For this review, take the finished solid that the model builds, in its own axes (mm). Face numbers are marked on the shaded views. A direction names the side the tool comes from. Coordinates: 2 decimals unless noted, no trailing zeros. Loops run counter-clockwise (first coordinate to the right, second up) from the corner with the lowest first, then second, coordinate; pieces in that order, holes last.
1. Take a section at A-A, the plane x = 1.5. State the section outline as (y, z) points, then the cut area to 3 significant figures.
2. Machinability: for the marked faces 4, 5 and 6, which of the approach directions +Z, -Z, +X, -X, +Y, -Y give a long, thin tool a straight path to every point of the face, cutting with its end or side? Answer none if there is none.
3. To check wall thickness, follow probe 1 along Z at (x, y) = (1.75, 0); probe 2 along Z at (x, y) = (3.75, 0); probe 3 along Y at (x, z) = (5.25, 2). State the ranges of each line that lie inside material, in increasing order.
4. Mouldability with a two-part tool opening along Y and no side actions: class the marked faces 1, 2 and 3 as pulls with the +Y half, pulls with the -Y half, needs draft (parallel to the pull), parting line crosses it, or undercut.
5. Clearance check with flat-ended pins moving along their axes: P1, Ø6, axis at x = 1, z = 11.5, coming from the -Y side; P2, Ø1.5, axis at x = -3.5, y = 13, coming from the -Z side; P3, Ø4, axis at x = 4.5, y = 12, coming from the -Z side; P4, Ø11, axis at y = -2.5, z = -0.5, coming from the -X side. State where each tip first meets the part, or that it passes through.
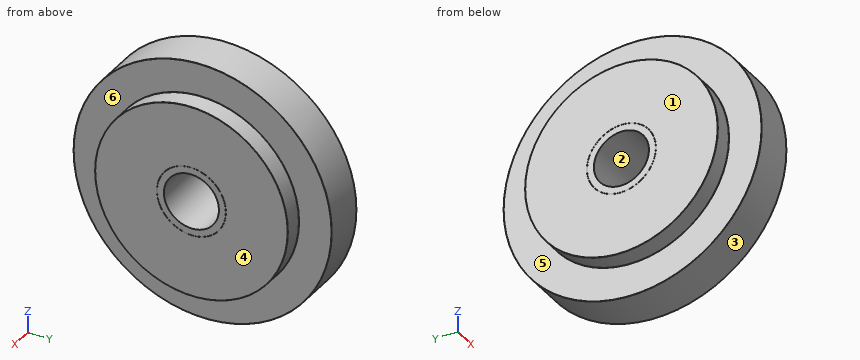
Autodesk Inventor part; units mm, degrees
ref_plane "to_bolt_XY" through (5.8, 0, 0) normal (1, 0, 0) x (0, 0, -1)
ref_plane "to_bolt_YZ" through (5.8, 0, 0) normal (0, 0, -1) x (0, 1, 0)
ref_plane "to_bolt_ZX" through (5.8, 0, 0) normal (0, 1, 0) x (1, 0, 0)
sketch "Sketch_1" plane through (0, 0, 0) normal (0, 0, 1) x (1, 0, 0)
  line L0 (5.8, 0) -> (-5.8, 0)
  line L1 (-5.8, 5.02) -> (-5.78, 5)
  line L2 (-5.78, 5) -> (5.78, 5)
  line L3 (5.78, 5) -> (5.8, 5.02)
  line L4 (5.8, 5.02) -> (5.8, 13.98)
  line L5 (5.8, 13.98) -> (5.78, 14)
  line L6 (5.78, 14) -> (3.081, 14)
  arc A0 (3.05, 14.031) -> (3.081, 14) centre (3.081, 14.031) ccw
  line L7 (3.05, 14.031) -> (3.05, 18.73)
  line L8 (3.05, 18.73) -> (3.03, 18.75)
  line L9 (3.03, 18.75) -> (-3.03, 18.75)
  line L10 (-3.03, 18.75) -> (-3.05, 18.73)
  line L11 (-3.05, 18.73) -> (-3.05, 14.031)
  arc A1 (-3.081, 14) -> (-3.05, 14.031) centre (-3.081, 14.031) ccw
  line L12 (-3.081, 14) -> (-5.78, 14)
  line L13 (-5.78, 14) -> (-5.8, 13.98)
  line L14 (-5.8, 13.98) -> (-5.8, 5.02)
revolve "Revolution1" add sketch "Sketch_1" angle 360 about axis through (5.8, 0, 0) along (1, 0, 0)
sketch "Sketch_2" plane through (0, 0, 0) normal (0, 0, 1) x (1, 0, 0)
  line L0 (5.8, 0) -> (-5.8, 0)
  line L1 (-5.8, 5) -> (-5.8, 4)
  line L2 (-5.8, 4) -> (5.8, 4)
  line L3 (5.8, 4) -> (5.8, 5)
  line L4 (5.8, 5) -> (-5.8, 5)
revolve "Revolution2" add sketch "Sketch_2" angle 360 about axis through (5.8, 0, 0) along (1, 0, 0)
ref_plane "to_bolt_XY" through (5.8, 0, 0) normal (1, 0, 0) x (0, 0, -1)
ref_plane "to_bolt_YZ" through (5.8, 0, 0) normal (0, 0, -1) x (0, 1, 0)
ref_plane "to_bolt_ZX" through (5.8, 0, 0) normal (0, 1, 0) x (1, 0, 0)
ref_plane "wheel_XY" through (0, 0, 0) normal (1, 0, 0) x (0, 0, -1)
ref_plane "wheel_YZ" through (0, 0, 0) normal (0, 0, -1) x (0, 1, 0)
ref_plane "wheel_ZX" through (0, 0, 0) normal (0, 1, 0) x (1, 0, 0)
properties part number "25-2281_w"
Results list:
1. outline: circle Ø37.5 at (0, 0); hole circle Ø8 at (0, 0)
1. area: 1,050 mm2
2. face 4: +Z, -Z, +X, +Y, -Y
2. face 5: -X
2. face 6: +X
3. probe 1: z = -18.75 to -4, 4 to 18.75
3. probe 2: z = -14 to -4, 4 to 14
3. probe 3: y = -13.86 to -3.46, 3.46 to 13.86
4. face 1: needs draft
4. face 2: undercut
4. face 3: parting line crosses it
5. P1: stops at y = -16.71
5. P2: stops at z = -14.05
5. P3: stops at z = -15.44
5. P4: stops at x = -5.8
